Drawing for the job (mm, zero at the part's lowest x, y, z). A direction names the side the tool comes from. Coordinates: 2 decimals unless noted, no trailing zeros. Write each loop counter-clockwise with the first axis right and the second up, starting at its lowest first coordinate (ties: lowest second). Pieces come first, ordered by that corner, then holes. Notation, with made-up numbers: (28.5, 74.5) -> (58.5, 74.5) arc R33 ccw to (58.5, 112.5) -> close; hole circle Ø9 at (68.5, 41.5). An arc over 180 degrees is marked (long way). Write item = value, one per line. Start each with the question number.
Q1. Band-saw the part on B-B, the plane z = 8.5. List the corners of the cut face in (x, y).
Q2. Band-saw the part on C-C, the plane y = 14. List the corners of the cut face in (x, z), plus the area to 3 significant figures.
Q3. Tool access for the marked faces 1 and 2: list every direction of +Z, -Z, +X, -X, +Y, -Y with a clear straight run to the whole face (end or side of a thin tool).
Q4. Band-saw the part on A-A, the plane x = 20. List the corners of the cut face in (y, z).
Q5. Pin check, flat tips, straight feed: P1, Ø6, axis at x = 55, z = 11, coming from the -Y side; P2, Ø3, axis at x = 20, z = 8.5, coming from the -Y side; P3, Ø4, axis at x = 17, y = 33.5, coming from the +Z side. Stop position of each tip, or through.
Q6. Probe line 1 (X direction, y = 39, z = 8.5); line 2 (Y direction, x = 46, z = 12); line 3 (Z direction, x = 7, y = 19). List the from-to ranges inside material, lowest first.
Q7. Band-saw the part on D-D, the plane x = 60. List the corners of the cut face in (y, z), plus the area to 3 significant figures.
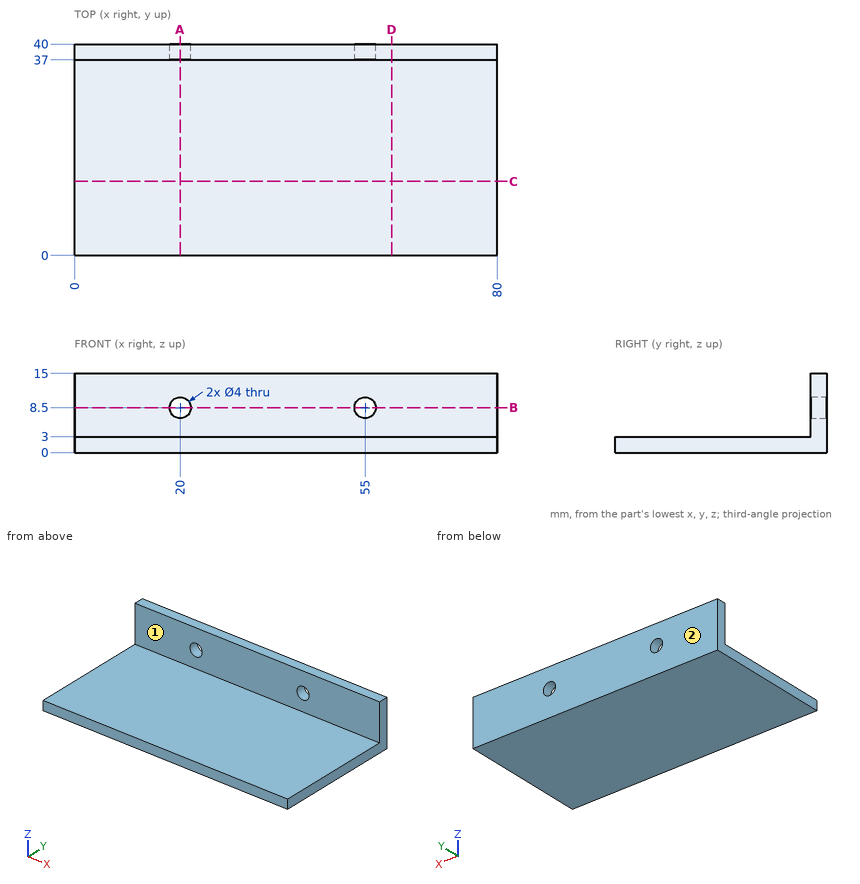
Ans:
q1.outline = (0, 37) -> (18, 37) -> (18, 40) -> (0, 40) -> close; (22, 37) -> (53, 37) -> (53, 40) -> (22, 40) -> close; (57, 37) -> (80, 37) -> (80, 40) -> (57, 40) -> close
q2.outline = (0, 0) -> (80, 0) -> (80, 3) -> (0, 3) -> close
q2.area = 240 mm2
q3.face_1 = +Z, +X, -X, -Y
q3.face_2 = +Z, -Z, +X, -X, +Y
q4.outline = (0, 0) -> (40, 0) -> (40, 6.5) -> (37, 6.5) -> (37, 3) -> (0, 3) -> close; (37, 10.5) -> (40, 10.5) -> (40, 15) -> (37, 15) -> close
q5.P1 = 37
q5.P2 = through
q5.P3 = 3
q6.line_1 = 0 to 18, 22 to 53, 57 to 80
q6.line_2 = 37 to 40
q6.line_3 = 0 to 3
q7.outline = (0, 0) -> (40, 0) -> (40, 15) -> (37, 15) -> (37, 3) -> (0, 3) -> close
q7.area = 156 mm2
